Part model, mm, in its own coordinate system. Round coordinates to 2 decimals unless told otherwise and drop trailing zeros. Return JSON: item names as keys, results as strings. Group by question number.
Item 1: Probe probe 1 along Y at (x, z) = (-80, 2.1); probe 2 along Y at (x, z) = (-69, 1.9). List the from-to ranges inside material, lowest first.
Item 2: Drop flat-ended pins along their axis: pin 1 (4 mm diameter, centred on x = -80.95, y = 0, fed in from -Z); pin 2 (4.5 mm diameter, centred on x = 59.05, y = 0, fed in from -Z); pin 3 (3 mm diameter, centred on x = 69.05, y = 0, fed in from +Z). Give the stop position or say it passes through.
Item 3: Saw through at A-A on z = 1.2. State how many separate pieces and enclosed holes the cut face has, and give its area (3 significant figures).
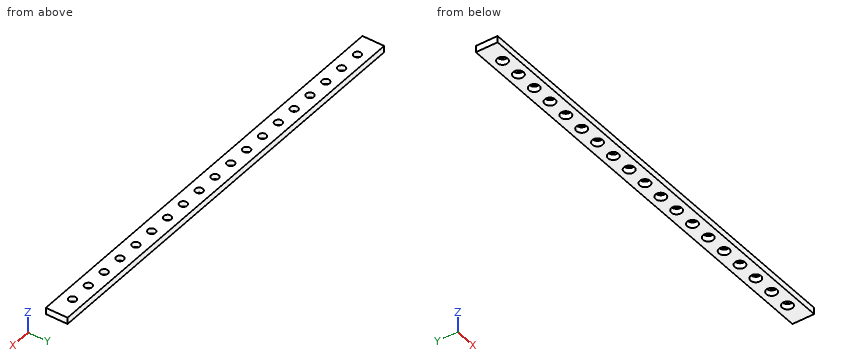
```python
from build123d import *

# Parameters (mm, degrees)
F0_W     = 200
F0_H     = 10
F1_DEPTH = 3
F2_D     = 4.8
F2_DEPTH = 2.6
F2_TIP   = 1.4420654857


with BuildPart() as f1:
    # F0 (on Top) → F1 (new body)
    with BuildSketch(Plane.XY):
        with Locations((-0.9545272589, 0)):
            Rectangle(F0_W, F0_H)
    extrude(amount=F1_DEPTH)

    # F2
    with Locations(Plane(origin=(0, 0, 0), x_dir=(1, 0, 0), z_dir=(0, 0, -1))):
        with Locations((-90.9545272589, 0), (-80.9545272589, 0), (-70.9545272589, 0), (-60.9545272589, 0), (-50.9545272589, 0), (-40.9545272589, 0), (-30.9545272589, 0), (-20.9545272589, 0), (-10.9545272589, 0), (-0.9545272589, 0), (9.0454727411, 0), (19.0454727411, 0), (29.0454727411, 0), (39.0454727411, 0), (49.0454727411, 0), (59.0454727411, 0), (69.0454727411, 0), (79.0454727411, 0), (89.0454727411, 0)):
            Hole(F2_D / 2, depth=F2_DEPTH)
            with Locations((0, 0, -(F2_DEPTH + F2_TIP / 2))):  # 118° drill point
                Cone(0, F2_D / 2, F2_TIP, mode=Mode.SUBTRACT)


solid = f1.part
```
Filled in:
{
 "1": {"probe 1": "y = -5 to -2.2, 2.2 to 5", "probe 2": "y = -5 to -1.39, 1.39 to 5"},
 "2": {"pin 1": "stops at z = 2.84", "pin 2": "stops at z = 2.69", "pin 3": "passes through"},
 "3": {"separate pieces": "1", "enclosed holes": "19", "area": "1,660 mm^2"}
}
